Part model, mm, in its own coordinate system. A direction names the side the tool comes from. Give positions to 0.01 mm unless a question says otherwise; leave off trailing zeros. Order: outer loops, then holes, each group sorted by start corner. A loop starts at its lowest first (then second) coordinate and runs counter-clockwise, first axis right, second up. Notation, with made-up numbers: (-24, -32) - (-11, -32) arc R9 ccw to (-11, -26) - close; hole circle Ø2 at (-17.5, 20.25). An arc over 180 degrees is marked (long way). One line per item, written item: value.
```python
from build123d import *

# Parameters (mm, degrees)
F1_DEPTH  = 258
F2_R      = 22.5
F2_R_2    = 3.25
F3_DEPTH  = 180.001
F2_R_3    = 5
F4_DEPTH  = 4
F5_R      = 4
F6_DEPTH  = 100.001
F7_R      = 3
F8_DEPTH  = 180.001
F9_SIZE2  = 3
F9_SIZE   = 3
F10_R     = 34.5
F10_R_2   = 19
F11_DEPTH = 9
F12_SIZE  = 1


with BuildPart() as f1:
    # F0 (on Front) → F1 (new body)
    with BuildSketch(Plane.XZ):
        with BuildLine():
            Line((0, 4), (0, 0))
            Line((0, 0), (96, 0))
            ThreePointArc((96, 0), (98.8284271247, 1.1715728753), (100, 4))
            Line((100, 4), (100, 176))
            ThreePointArc((100, 176), (98.8284271247, 178.8284271247), (96, 180))
            Line((96, 180), (0, 180))
            Line((0, 180), (0, 176))
            Line((0, 176), (94, 176))
            ThreePointArc((94, 176), (95.4142135624, 175.4142135624), (96, 174))
            Line((96, 174), (96, 6))
            ThreePointArc((96, 6), (95.4142135624, 4.5857864376), (94, 4))
            Line((94, 4), (0, 4))
        make_face()
    extrude(amount=F1_DEPTH)

    # F2 (on face) → F3 (cut, through all)
    with BuildSketch(Plane.XY.offset(180)):
        with Locations((50, -200.5)):
            Circle(F2_R)
        with Locations((50, -87.5)):
            Circle(F2_R_2)
        with Locations((50, -57.5)):
            Circle(F2_R)
        with Locations((20, -57.5)):
            Circle(F2_R_2)
        with Locations((80, -57.5)):
            Circle(F2_R_2)
        with Locations((50, -27.5)):
            Circle(F2_R_2)
        with Locations((50, -170.5)):
            Circle(F2_R_2)
        with Locations((80, -200.5)):
            Circle(F2_R_2)
        with Locations((50, -230.5)):
            Circle(F2_R_2)
        with Locations((20, -200.5)):
            Circle(F2_R_2)
    extrude(amount=-F3_DEPTH, mode=Mode.SUBTRACT)

    # F2 (on face) → F4 (cut, through all)
    with BuildSketch(Plane.XY.offset(180)):
        with Locations((50, -129)):
            Circle(F2_R_3)
    extrude(amount=-F4_DEPTH, mode=Mode.SUBTRACT)

    # F5 (on face) → F6 (cut, through all)
    with BuildSketch(Plane.YZ.offset(100)):
        with Locations((-233.5, 148.5)):
            Circle(F5_R)
        with Locations((-233.5, 31.5)):
            Circle(F5_R)
        with Locations((-157.5, 148.5)):
            Circle(F5_R)
        with Locations((-157.5, 31.5)):
            Circle(F5_R)
        with Locations((-100.5, 148.5)):
            Circle(F5_R)
        with Locations((-100.5, 31.5)):
            Circle(F5_R)
        with Locations((-24.5, 148.5)):
            Circle(F5_R)
        with Locations((-24.5, 31.5)):
            Circle(F5_R)
    extrude(amount=-F6_DEPTH, mode=Mode.SUBTRACT)

    # F7 (on face) → F8 (cut, through all)
    with BuildSketch(Plane.XY.offset(180)):
        with Locations((10, -239)):
            Circle(F7_R)
        with Locations((10, -19)):
            Circle(F7_R)
    extrude(amount=-F8_DEPTH, mode=Mode.SUBTRACT)

    # F9
    f9_edges = [f1.edges().sort_by_distance(p)[0] for p in [
        (7, -19, 180),
        (7, -239, 180),
        (7, -239, 0),
        (7, -19, 0),
    ]]
    chamfer(f9_edges, length=F9_SIZE, length2=F9_SIZE2)

    # F10 (on face) → F11 (join)
    with BuildSketch(Plane(origin=(0, 0, 0), x_dir=(1, 0, 0), z_dir=(0, 0, -1))):
        with Locations((50, 57.5)):
            Circle(F10_R)
        with Locations((50, 57.5)):
            Circle(F10_R_2, mode=Mode.SUBTRACT)
        with Locations((50, 200.5)):
            Circle(F10_R)
        with Locations((50, 200.5)):
            Circle(F10_R_2, mode=Mode.SUBTRACT)
    extrude(amount=F11_DEPTH)

    # F12
    f12_edges = [f1.edges().sort_by_distance(p)[0] for p in [
        (15.5, -200.5, -9),
        (15.5, -57.5, -9),
    ]]
    chamfer(f12_edges, length=F12_SIZE)


solid = f1.part
```
1) Drill centre lines: line 1 along Y through (x, z) = (10, 3); line 2 along Z through (x, y) = (44.5, -172); line 3 along Z through (x, y) = (93.5, -55). Where is each one in solid material? Low to high. Write a range as from..to.
Outcome:
line 1: y = -258..-242, -236..-22, -16..0
line 2: z = -9..4, 176..180
line 3: z = 0..4, 176..180
2) Mould opens along X. For faces 4 (the cylindrical face through (98.028, -153.685, 32.701)), 5 (the flat face through (100, -127, 89)), 6 (the flat face through (96, -127, 91)), 7 (the flat face through (80, -58, 0)) say: released by +X, released by -X, zero draft, split by the parting line, or undercut.
Outcome:
face 4: zero draft
face 5: released by +X
face 6: released by -X
face 7: undercut
3) Cut at B-B, the plane y = -129. Give the cut face in (x, z).
Outcome:
outline: (0, 0) - (96, 0) arc R4 ccw to (100, 4) - (100, 176) arc R4 ccw to (96, 180) - (55, 180) - (55, 176) - (94, 176) arc R2 cw to (96, 174) - (96, 6) arc R2 cw to (94, 4) - (0, 4) - close; (0, 176) - (45, 176) - (45, 180) - (0, 180) - close
4) Cut at C-C, the plane x = 50. Give the number of separate pieces and of enclosed holes in the cut face, then the cut area to 3 significant figures.
Outcome:
separate pieces: 11
enclosed holes: 0
area: 1,650 mm^2
5) Pin check, flat tips, straight feed: pin 1 (3 mm diameter, centred on x = 78.5, y = -200, fed in from +Z); pin 2 (13 mm diameter, centred on y = -100.5, z = 148.5, fed in from -X); pin 3 (9 mm diameter, centred on y = -24.5, z = 31.5, fed in from +X); pin 4 (6 mm diameter, centred on x = 27.5, y = -112.5, fed in from -Z). Stop position of each tip, or through.
Outcome:
pin 1: stops at z = 0
pin 2: stops at x = 96
pin 3: stops at x = 100
pin 4: stops at z = 0
6) Which spindle directions (+Z, -Z, +X, -X, +Y, -Y) get a long thin tool onto all of the face, cutting with end or side? Do faces 1 (the cylindrical face through (98.028, -101.021, 152.466)), 2 (the cylindrical face through (53.002, -28.745, 178.028)), 3 (the flat face through (48, -127, 4)). Say none if no direction does.
Outcome:
face 1: +X, -X
face 2: +Z
face 3: -X, +Y, -Y
7) Cut at A-A, the plane y = -157.5. Give the cut face in (x, z).
Outcome:
outline: (0, 0) - (96, 0) arc R4 ccw to (100, 4) - (100, 27.5) - (96, 27.5) - (96, 6) arc R2 cw to (94, 4) - (0, 4) - close; (0, 176) - (94, 176) arc R2 cw to (96, 174) - (96, 152.5) - (100, 152.5) - (100, 176) arc R4 ccw to (96, 180) - (0, 180) - close; (96, 35.5) - (100, 35.5) - (100, 144.5) - (96, 144.5) - close
